```python
from build123d import *

# Parameters (mm, degrees)
SKETCH1_W           = 149.86
SKETCH1_H           = 76.2
SKETCH1_W_2         = 19.05
SKETCH1_H_2         = 6.35
BOSS_EXTRUDE1_DEPTH = 6.35
SKETCH2_W           = 6.35
SKETCH2_H           = 9.525
SKETCH2_W_2         = 9.525
SKETCH2_H_2         = 6.35
SKETCH2_W_3         = 6.985
BOSS_EXTRUDE2_DEPTH = 6.35


with BuildPart() as part:
    # Sketch1 → Boss-Extrude1 (new body)
    with BuildSketch(Plane(origin=(0, 0, 0), x_dir=(1, 0, 0), z_dir=(0, 1, 0))):
        with Locations((74.93, -38.1)):
            Rectangle(SKETCH1_W, SKETCH1_H)
        with Locations((15.875, -66.675)):
            Rectangle(SKETCH1_W_2, SKETCH1_H_2, mode=Mode.SUBTRACT)
        with Locations((15.875, -9.525)):
            Rectangle(SKETCH1_W_2, SKETCH1_H_2, mode=Mode.SUBTRACT)
        with Locations((133.985, -66.675)):
            Rectangle(SKETCH1_W_2, SKETCH1_H_2, mode=Mode.SUBTRACT)
        with Locations((133.985, -9.525)):
            Rectangle(SKETCH1_W_2, SKETCH1_H_2, mode=Mode.SUBTRACT)
    extrude(amount=BOSS_EXTRUDE1_DEPTH)

    # Sketch2 → Boss-Extrude2 (add)
    with BuildSketch(Plane.XZ):
        with Locations((-3.175, 52.3875)):
            Rectangle(SKETCH2_W, SKETCH2_H)
        with Locations((-3.175, 33.3375)):
            Rectangle(SKETCH2_W, SKETCH2_H)
        with Locations((14.2875, -3.175)):
            Rectangle(SKETCH2_W_2, SKETCH2_H_2)
        with Locations((52.3875, -3.175)):
            Rectangle(SKETCH2_W_2, SKETCH2_H_2)
        with Locations((71.4375, -3.175)):
            Rectangle(SKETCH2_W_2, SKETCH2_H_2)
        with Locations((90.4875, -3.175)):
            Rectangle(SKETCH2_W_2, SKETCH2_H_2)
        with Locations((128.5875, -3.175)):
            Rectangle(SKETCH2_W_2, SKETCH2_H_2)
        with Locations((146.3675, -3.175)):
            Rectangle(SKETCH2_W_3, SKETCH2_H_2)
        with Locations((153.035, 42.8625)):
            Rectangle(SKETCH2_W, SKETCH2_H)
        Polygon((142.875, 82.55), (142.875, 76.2), (149.86, 76.2), (152.4, 76.2), (152.4, 82.55), align=None)
        with Locations((109.5375, 79.375)):
            Rectangle(SKETCH2_W_2, SKETCH2_H_2)
        with Locations((90.4875, 79.375)):
            Rectangle(SKETCH2_W_2, SKETCH2_H_2)
        with Locations((33.3375, 79.375)):
            Rectangle(SKETCH2_W_2, SKETCH2_H_2)
        with Locations((14.2875, 79.375)):
            Rectangle(SKETCH2_W_2, SKETCH2_H_2)
        with Locations((128.5875, 79.375)):
            Rectangle(SKETCH2_W_2, SKETCH2_H_2)
        with Locations((-3.175, 71.4375)):
            Rectangle(SKETCH2_W, SKETCH2_H)
        with Locations((-3.175, 14.2875)):
            Rectangle(SKETCH2_W, SKETCH2_H)
        with Locations((33.3375, -3.175)):
            Rectangle(SKETCH2_W_2, SKETCH2_H_2)
        with Locations((109.5375, -3.175)):
            Rectangle(SKETCH2_W_2, SKETCH2_H_2)
        with Locations((153.035, 4.7625)):
            Rectangle(SKETCH2_W, SKETCH2_H)
        with Locations((153.035, 23.8125)):
            Rectangle(SKETCH2_W, SKETCH2_H)
        with Locations((153.035, 61.9125)):
            Rectangle(SKETCH2_W, SKETCH2_H)
        with Locations((71.4375, 79.375)):
            Rectangle(SKETCH2_W_2, SKETCH2_H_2)
        with Locations((52.3875, 79.375)):
            Rectangle(SKETCH2_W_2, SKETCH2_H_2)
    extrude(amount=-BOSS_EXTRUDE2_DEPTH)


solid = part.part
```
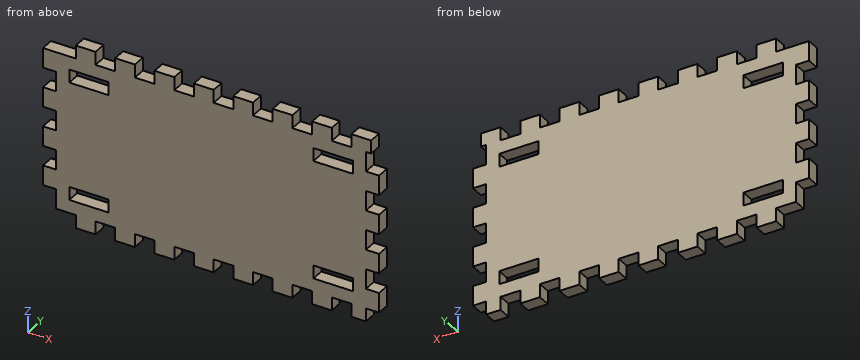
Here's how the part is built. I have some questions about the finished solid (model axes, mm). Give positions to 0.01 mm unless a question says otherwise; leave off trailing zeros. Write each loop counter-clockwise with the first axis right and the second up, starting at its lowest first coordinate (ties: lowest second). Pieces come first, ordered by that corner, then holes.
(1) Imagine slicing it at A-A, the plane x = 13. Write out the boundary of the cut face in (y, z).
Output values:
outline: (0, -6.35) - (6.35, -6.35) - (6.35, 6.35) - (0, 6.35) - close; (0, 12.7) - (6.35, 12.7) - (6.35, 63.5) - (0, 63.5) - close; (0, 69.85) - (6.35, 69.85) - (6.35, 82.55) - (0, 82.55) - close
(2) Imagine slicing it at C-C, the plane y = 4.5. Count the separate pieces of the cut face and the enclosed holes in it, and give its area (3 significant figures).
Output values:
separate pieces: 1
enclosed holes: 4
area: 12,400 mm2
(3) Imagine slicing it at D-D, the plane x = 79. Write out the boundary of the cut face in (y, z).
Output values:
outline: (0, 0) - (6.35, 0) - (6.35, 76.2) - (0, 76.2) - close
(4) Imagine slicing it at B-B, the plane z = 15.5. Write out the boundary of the cut face in (x, y).
Output values:
outline: (-6.35, 0) - (149.86, 0) - (149.86, 6.35) - (-6.35, 6.35) - close
(5) If I drill on L1, parallel to Z at x = 136, y = 5.75; L2, parallel to X at y = 4, z = 12; L3, parallel to Z at x = 41, y = 3.75, over which ranges is the centre line in solid material (lowest first)?
Output values:
L1: z = 0 to 6.35, 12.7 to 63.5, 69.85 to 76.2
L2: x = -6.35 to 6.35, 25.4 to 124.46, 143.51 to 149.86
L3: z = 0 to 76.2
(6) Will these pins go through, and if not, where does the flat tip stop? pin 1 (3 mm diameter, centred on y = 4, z = 14, fed in from +X); pin 2 (1.9 mm diameter, centred on x = -4.5, y = 2.5, fed in from -Z) (3 decimals); pin 3 (1.9 mm diameter, centred on x = 153.5, y = 3.5, fed in from -Z).
Output values:
pin 1: stops at x = 149.86
pin 2: stops at z = 9.525
pin 3: stops at z = 0
